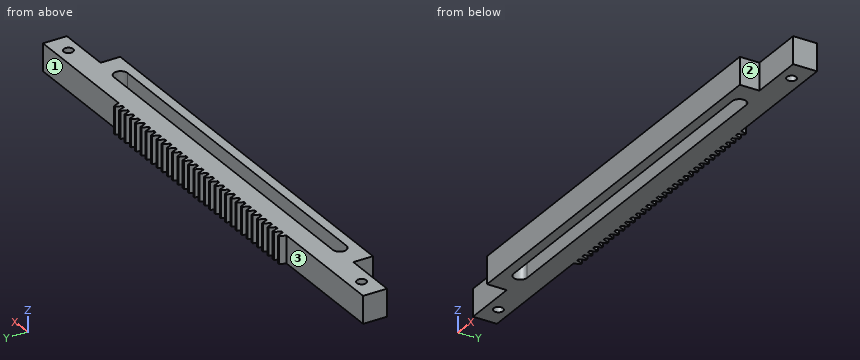
from build123d import *

# Parameters (mm, degrees)
BLANKSKE_W          = 100
BLANKSKE_H          = 11
BLANK_DEPTH         = 10
TOOTHCUTSIM_DEPTH   = 102.098961419
TEETHCUTS_COUNT     = 33
TEETHCUTS_PITCH     = 3.14159265
SKETCH1_W           = 10
SKETCH1_H           = 8.987737656
BOSS_EXTRUDE1_DEPTH = 45
SKETCH2_W           = 10
SKETCH2_H           = 8.75
BOSS_EXTRUDE2_DEPTH = 45
SKETCH3_R           = 1.75
CUT_EXTRUDE1_DEPTH  = 146.760076839
SKETCH4_W           = 150
SKETCH4_H           = 10
BOSS_EXTRUDE3_DEPTH = 7.2
CUT_EXTRUDE2_DEPTH  = 146.760076839
CUT_EXTRUDE3_DEPTH  = 146.760076839


with BuildPart() as part:
    # BlankSke → Blank (new body)
    with BuildSketch(Plane.XY):
        with Locations((50, 5.5)):
            Rectangle(BLANKSKE_W, BLANKSKE_H)
    extrude(amount=-BLANK_DEPTH)

    # TooCutSkeSim → ToothCutSim (cut, through all)
    with BuildSketch(Plane.XY):
        Polygon((0.44443537, 8.75), (-0.44443537, 8.75), (-1.272613241, 11.0254), (1.272613241, 11.0254), align=None)
    toothcutsim = extrude(amount=-TOOTHCUTSIM_DEPTH, mode=Mode.SUBTRACT)

    # TeethCuts: ToothCutSim ×33
    with Locations(*[(i * TEETHCUTS_PITCH, 0, 0) for i in range(1, TEETHCUTS_COUNT)]):
        add(toothcutsim, mode=Mode.SUBTRACT)

    # Sketch1 → Boss-Extrude1 (add)
    with BuildSketch(Plane(origin=(100, 0, 0), x_dir=(0, 0, -1), z_dir=(1, 0, 0))):
        with Locations((5, 4.493868828)):
            Rectangle(SKETCH1_W, SKETCH1_H)
    extrude(amount=BOSS_EXTRUDE1_DEPTH)

    # Sketch2 → Boss-Extrude2 (add)
    with BuildSketch(Plane.ZY):
        with Locations((-5, 4.375)):
            Rectangle(SKETCH2_W, SKETCH2_H)
    extrude(amount=BOSS_EXTRUDE2_DEPTH)

    # Sketch3 → Cut-Extrude1 (cut, through all)
    with BuildSketch(Plane(origin=(0, 0, -10), x_dir=(-1, 0, 0), z_dir=(0, 0, -1))):
        with Locations((-137, 4.375)):
            Circle(SKETCH3_R)
        with Locations((37, 4.375)):
            Circle(SKETCH3_R)
    extrude(amount=-CUT_EXTRUDE1_DEPTH, mode=Mode.SUBTRACT)

    # Sketch4 → Boss-Extrude3 (add)
    with BuildSketch(Plane.XZ):
        with Locations((50, -5)):
            Rectangle(SKETCH4_W, SKETCH4_H)
    extrude(amount=BOSS_EXTRUDE3_DEPTH)

    # Sketch5 → Cut-Extrude2 (cut, through all)
    with BuildSketch(Plane.XY):
        with BuildLine():
            Line((-15, 1.3), (115, 1.3))
            ThreePointArc((115, 1.3), (117.5, -1.2), (115, -3.7))
            Line((115, -3.7), (-15, -3.7))
            ThreePointArc((-15, -3.7), (-17.5, -1.2), (-15, 1.3))
        make_face()
    extrude(amount=-CUT_EXTRUDE2_DEPTH, mode=Mode.SUBTRACT)

    # Sketch6 → Cut-Extrude3 (cut, through all)
    with BuildSketch(Plane.XY):
        Polygon((100, 8.987737656), (100.08652943, 8.75), (145, 8.75), (145, 8.987737656), align=None)
    extrude(amount=-CUT_EXTRUDE3_DEPTH, mode=Mode.SUBTRACT)


solid = part.part
Here's how the part is built. I have some questions about the finished solid (model axes, mm). Face numbers are marked on the shaded views. A direction names the side the tool comes from. Round coordinates to 2 decimals unless told otherwise and drop trailing zeros. Order: outer loops, then holes, each group sorted by start corner. A loop starts at its lowest first (then second) coordinate and runs counter-clockwise, first axis right, second up. Notation, with made-up numbers: (81, -16.5) -> (127, -16.5) arc R18 cw to (127, 1.5) -> close; hole circle Ø1 at (26.5, 45). An arc over 180 degrees is marked (long way). Return JSON: item names as keys, results as strings.
Q1. For pin 1 Ø3 at (y, z) = (-3.5, -7) entering from -X; pin 2 Ø5 at (x, y) = (122, 8.5) entering from +Z; pin 3 Ø0.7 at (x, z) = (66, -7.5) entering from +Y; pin 4 Ø3 at (y, z) = (-2.5, -4.5) entering from +X, each with a flat end and sliding along its axis, tell me the tip position at first contact or that it passes through.
Filled sheet:
{"pin 1": "stops at x = -25", "pin 2": "stops at z = 0", "pin 3": "stops at y = 8.75", "pin 4": "stops at x = 125"}
Q2. Which directions (+Z, -Z, +X, -X, +Y, -Y) give clear straight access to the entire face, cutting with the end or side of a thin tool? Please do the marked faces 1, 2 and 3.
Filled sheet:
{"face 1": "+Z, -Z, +X, +Y", "face 2": "+Z, -Z, +X, -Y", "face 3": "+Z, -Z, -X, +Y"}
Q3. If we section it at B-B on y = -5.25: List the corners of the cut face in (x, z) for me, plus the area to 3 significant figures.
Filled sheet:
{"outline": "(-25, -10) -> (125, -10) -> (125, 0) -> (-25, 0) -> close", "area": "1,500 mm^2"}
Q4. If we section it at C-C on z = -3.5: Give the number of separate pieces and of enclosed holes in the cut face, plus the area to 3 significant figures.
Filled sheet:
{"separate pieces": "1", "enclosed holes": "3", "area": "2,160 mm^2"}
Q5. If we section it at A-A on x = -37: List the corners of the cut face in (y, z) for me (3 decimals), plus the area to 3 significant figures.
Filled sheet:
{"outline": "(0, -10) -> (2.625, -10) -> (2.625, 0) -> (0, 0) -> close; (6.125, -10) -> (8.75, -10) -> (8.75, 0) -> (6.125, 0) -> close", "area": "52.5 mm^2"}
Q6. I need wall thicknesses on line 1 along Y through (x, z) = (-37, -5.5) (3 decimals); line 2 along Y through (x, z) = (-9, -3); line 3 along X through (y, z) = (5.5, -2). Which ranges of each line are inside material? Lowest first, please. Write a range as from..to.
Filled sheet:
{"line 1": "y = 0..2.625, 6.125..8.75", "line 2": "y = -7.2..-3.7, 1.3..8.75", "line 3": "x = -45..-38.34, -35.66..135.66, 138.34..145"}
